Part model, mm, in its own coordinate system. Give positions to 0.01 mm unless a question says otherwise; leave off trailing zeros. Write each loop counter-clockwise with the first axis right and the second up, starting at its lowest first coordinate (ties: lowest second). Pieces come first, ordered by that corner, then holes.
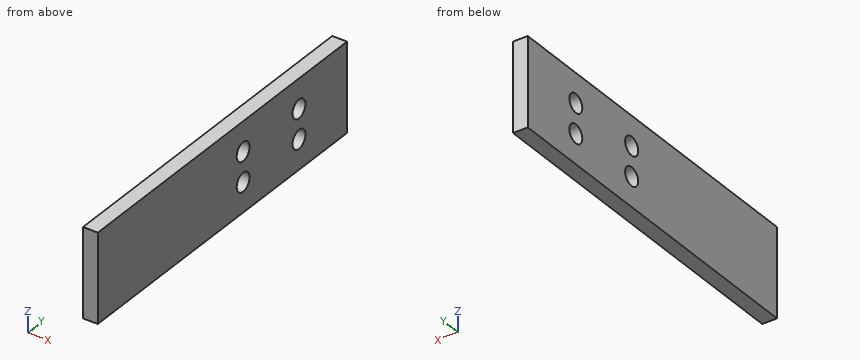
from build123d import *

# Parameters (mm, degrees)
F0_W     = 3.175
F0_H     = 19.05
F1_DEPTH = 38.1
F2_R     = 1.9812
F3_DEPTH = 3.176
F4_R     = 1.9812
F5_DEPTH = 3.176


with BuildPart() as f1:
    # F0 (on Front) → F1 (new body, symmetric)
    with BuildSketch(Plane.XZ):
        Rectangle(F0_W, F0_H)
    extrude(amount=F1_DEPTH, both=True)

    # F2 (on face) → F3 (cut, through all)
    with BuildSketch(Plane.YZ.offset(1.5875)):
        with Locations((23.4188, 3.175)):
            Circle(F2_R)
        with Locations((23.4188, -3.175)):
            Circle(F2_R)
    extrude(amount=-F3_DEPTH, mode=Mode.SUBTRACT)

    # F4 (on face) → F5 (cut, through all)
    with BuildSketch(Plane.YZ.offset(1.5875)):
        with Locations((6.35, 3.175)):
            Circle(F4_R)
        with Locations((6.35, -3.175)):
            Circle(F4_R)
    extrude(amount=-F5_DEPTH, mode=Mode.SUBTRACT)


solid = f1.part
1) Drill centre lines: L1, parallel to Z at x = 0.3, y = 6.35 (3 decimals); L2, parallel to Y at x = 0.6, z = 3; L3, parallel to Y at x = -0.75, z = -2.25. Where is each one in solid material? Low to high.
Check result:
L1: z = -9.525 to -5.156, -1.194 to 1.194, 5.156 to 9.525
L2: y = -38.1 to 4.38, 8.32 to 21.45, 25.39 to 38.1
L3: y = -38.1 to 4.6, 8.1 to 21.67, 25.17 to 38.1
2) Saw through at A-A (y = 6.35). Write the cut outline in (x, z) (1 decimal).
Check result:
outline: (-1.6, -9.5) - (1.6, -9.5) - (1.6, -5.2) - (-1.6, -5.2) - close; (-1.6, -1.2) - (1.6, -1.2) - (1.6, 1.2) - (-1.6, 1.2) - close; (-1.6, 5.2) - (1.6, 5.2) - (1.6, 9.5) - (-1.6, 9.5) - close
3) Saw through at C-C (x = 0.2). Write the cut outline in (y, z) (3 decimals), and give its area (3 significant figures).
Check result:
outline: (-38.1, -9.525) - (38.1, -9.525) - (38.1, 9.525) - (-38.1, 9.525) - close; hole circle Ø3.962 at (6.35, -3.175); hole circle Ø3.962 at (6.35, 3.175); hole circle Ø3.962 at (23.419, -3.175); hole circle Ø3.962 at (23.419, 3.175)
area: 1,400 mm2
4) Saw through at B-B (z = 4.5). Write the cut outline in (x, y), and give its area (3 significant figures).
Check result:
outline: (-1.59, -38.1) - (1.59, -38.1) - (1.59, 4.88) - (-1.59, 4.88) - close; (-1.59, 7.82) - (1.59, 7.82) - (1.59, 21.95) - (-1.59, 21.95) - close; (-1.59, 24.89) - (1.59, 24.89) - (1.59, 38.1) - (-1.59, 38.1) - close
area: 223 mm2
